from build123d import *

# Parameters (mm, degrees)
F1_DEPTH = 127


with BuildPart() as f1:
    # F0 (on Top) → F1 (new body)
    with BuildSketch(Plane.XY):
        with BuildLine():
            Line((-42.099868, 63.5), (-63.5, 63.5))
            Line((-63.5, 63.5), (-63.5, 42.099868))
            Line((-63.5, 42.099868), (-50.8, 42.099868))
            Line((-50.8, 42.099868), (-50.8, 29.399868))
            Line((-50.8, 29.399868), (-63.5, 29.399868))
            Line((-63.5, 29.399868), (-63.5, 6.35))
            Line((-63.5, 6.35), (-50.8, 6.35))
            ThreePointArc((-50.8, 6.35), (-35.688296, 0), (-50.8, -6.35))
            Line((-50.8, -6.35), (-63.5, -6.35))
            Line((-63.5, -6.35), (-63.5, -29.399868))
            Line((-63.5, -29.399868), (-50.8, -29.399868))
            Line((-50.8, -29.399868), (-50.8, -42.099868))
            Line((-50.8, -42.099868), (-63.5, -42.099868))
            Line((-63.5, -42.099868), (-63.5, -63.5))
            Line((-63.5, -63.5), (-42.099868, -63.5))
            Line((-42.099868, -63.5), (-42.099868, -50.8))
            Line((-42.099868, -50.8), (-29.399868, -50.8))
            Line((-29.399868, -50.8), (-29.399868, -63.5))
            Line((-29.399868, -63.5), (-6.35, -63.5))
            Line((-6.35, -63.5), (-6.35, -50.8))
            ThreePointArc((-6.35, -50.8), (0, -35.688296), (6.35, -50.8))
            Line((6.35, -50.8), (6.35, -63.5))
            Line((6.35, -63.5), (29.399868, -63.5))
            Line((29.399868, -63.5), (29.399868, -50.8))
            Line((29.399868, -50.8), (42.099868, -50.8))
            Line((42.099868, -50.8), (42.099868, -63.5))
            Line((42.099868, -63.5), (63.5, -63.5))
            Line((63.5, -63.5), (63.5, -42.099868))
            Line((63.5, -42.099868), (50.8, -42.099868))
            Line((50.8, -42.099868), (50.8, -29.399868))
            Line((50.8, -29.399868), (63.5, -29.399868))
            Line((63.5, -29.399868), (63.5, -6.35))
            Line((63.5, -6.35), (50.8, -6.35))
            ThreePointArc((50.8, -6.35), (35.688296, 0), (50.8, 6.35))
            Line((50.8, 6.35), (63.5, 6.35))
            Line((63.5, 6.35), (63.5, 29.399868))
            Line((63.5, 29.399868), (50.8, 29.399868))
            Line((50.8, 29.399868), (50.8, 42.099868))
            Line((50.8, 42.099868), (63.5, 42.099868))
            Line((63.5, 42.099868), (63.5, 63.5))
            Line((63.5, 63.5), (42.099868, 63.5))
            Line((42.099868, 63.5), (42.099868, 50.8))
            Line((42.099868, 50.8), (29.399868, 50.8))
            Line((29.399868, 50.8), (29.399868, 63.5))
            Line((29.399868, 63.5), (6.35, 63.5))
            Line((6.35, 63.5), (6.35, 50.8))
            ThreePointArc((6.35, 50.8), (0, 35.688296), (-6.35, 50.8))
            Line((-6.35, 50.8), (-6.35, 63.5))
            Line((-6.35, 63.5), (-29.399868, 63.5))
            Line((-29.399868, 63.5), (-29.399868, 50.8))
            Line((-29.399868, 50.8), (-42.099868, 50.8))
            Line((-42.099868, 50.8), (-42.099868, 63.5))
        make_face()
        with BuildLine():
            Line((-57.15, 23.049868), (-44.45, 23.049868))
            Line((-44.45, 23.049868), (-44.45, 44.45))
            Line((-44.45, 44.45), (-23.049868, 44.45))
            Line((-23.049868, 44.45), (-23.049868, 57.15))
            Line((-23.049868, 57.15), (-12.7, 57.15))
            Line((-12.7, 57.15), (-12.7, 53.002523))
            ThreePointArc((-12.7, 53.002523), (0, 29.338296), (12.7, 53.002523))
            Line((12.7, 53.002523), (12.7, 57.15))
            Line((12.7, 57.15), (23.049868, 57.15))
            Line((23.049868, 57.15), (23.049868, 44.45))
            Line((23.049868, 44.45), (44.45, 44.45))
            Line((44.45, 44.45), (44.45, 23.049868))
            Line((44.45, 23.049868), (57.15, 23.049868))
            Line((57.15, 23.049868), (57.15, 12.7))
            Line((57.15, 12.7), (53.002523, 12.7))
            ThreePointArc((53.002523, 12.7), (29.338296, 0), (53.002523, -12.7))
            Line((53.002523, -12.7), (57.15, -12.7))
            Line((57.15, -12.7), (57.15, -23.049868))
            Line((57.15, -23.049868), (44.45, -23.049868))
            Line((44.45, -23.049868), (44.45, -44.45))
            Line((44.45, -44.45), (23.049868, -44.45))
            Line((23.049868, -44.45), (23.049868, -57.15))
            Line((23.049868, -57.15), (12.7, -57.15))
            Line((12.7, -57.15), (12.7, -53.002523))
            ThreePointArc((12.7, -53.002523), (0, -29.338296), (-12.7, -53.002523))
            Line((-12.7, -53.002523), (-12.7, -57.15))
            Line((-12.7, -57.15), (-23.049868, -57.15))
            Line((-23.049868, -57.15), (-23.049868, -44.45))
            Line((-23.049868, -44.45), (-44.45, -44.45))
            Line((-44.45, -44.45), (-44.45, -23.049868))
            Line((-44.45, -23.049868), (-57.15, -23.049868))
            Line((-57.15, -23.049868), (-57.15, -12.7))
            Line((-57.15, -12.7), (-53.002523, -12.7))
            ThreePointArc((-53.002523, -12.7), (-29.338296, 0), (-53.002523, 12.7))
            Line((-53.002523, 12.7), (-57.15, 12.7))
            Line((-57.15, 12.7), (-57.15, 23.049868))
        make_face(mode=Mode.SUBTRACT)
    extrude(amount=F1_DEPTH)


solid = f1.part
Geometry check sheet. Reference: the model listing, model coordinates, mm. A direction names the side the tool comes from. Round coordinates to 2 decimals unless told otherwise and drop trailing zeros. Order: outer loops, then holes, each group sorted by start corner. A loop starts at its lowest first (then second) coordinate and runs counter-clockwise, first axis right, second up. Notation, with made-up numbers: (61, 50.5) -> (85, 50.5) arc R23 ccw to (85, 71.5) -> close; hole circle Ø3 at (55, 78.5). An arc over 180 degrees is marked (long way). Use one line per item in the form item = value.
1. Go/stop test with flat-tipped pins: pin 1 (6.5 mm diameter, centred on x = 36.5, z = 69, fed in from -Y); pin 2 (6.5 mm diameter, centred on x = 35.5, z = 67.5, fed in from +Y). Record where each tip stops, or that it passes through.
Working result:
pin_1 = -50.8
pin_2 = 50.8
2. Cross-section at B-B, the plane x = 0. Enter the section's corners in (y, z).
Working result:
outline = (-35.69, 0) -> (-29.34, 0) -> (-29.34, 127) -> (-35.69, 127) -> close; (29.34, 0) -> (35.69, 0) -> (35.69, 127) -> (29.34, 127) -> close
3. Mould release check, pull along X, two halves, no side actions. Record for faces 1 (the face through (63.5, 53, 63)), 2 (the face through (-33, 0, 0)), 3 (the face through (-63.5, 18, 63)), 4 (the face through (35.693, -0.292, 62.611)): pulls with the +X half, pulls with the -X half, needs draft (parallel to the pull), parting line crosses it, or undercut.
Working result:
face_1 = pulls with the +X half
face_2 = needs draft
face_3 = pulls with the -X half
face_4 = undercut
4. Set-up check for faces 5 (the face through (-57, -6.35, 63)), 6 (the face through (-63.5, 53, 63)), 7 (the face through (-53, 63.5, 63)), 8 (the face through (-51, 23.05, 63)), 9 (the face through (57, -29.4, 63)): record each of +Z, -Z, +X, -X, +Y, -Y from which the full face is reachable in a straight line by a thin tool's end or side.
Working result:
face_5 = +Z, -Z, -X
face_6 = +Z, -Z, -X, +Y, -Y
face_7 = +Z, -Z, +X, -X, +Y
face_8 = +Z, -Z
face_9 = +Z, -Z, +X
5. Scan lines: line 1 along X through (y, z) = (-57.5, 72); line 2 along X through (y, z) = (53, 66.5); line 3 along X through (y, z) = (37.5, 103.5). Record each from-to range of solid material in increasing order. Write a range as from..to.
Working result:
line_1 = -63.5..-42.1, -29.4..-6.35, 6.35..29.4, 42.1..63.5
line_2 = -63.5..-42.1, -29.4..-23.05, -12.7..-6.35, 6.35..12.7, 23.05..29.4, 42.1..63.5
line_3 = -50.8..-44.45, -13.5..-5.38, 5.38..13.5, 44.45..50.8
6. Cross-section at A-A, the plane y = -17. Enter the section's corners in (x, z).
Working result:
outline = (-63.5, 0) -> (-57.15, 0) -> (-57.15, 127) -> (-63.5, 127) -> close; (57.15, 0) -> (63.5, 0) -> (63.5, 127) -> (57.15, 127) -> close
